Check sheet for the modelled part. Datum: model origin and axes. Units: mm. Round coordinates to 2 decimals unless told otherwise and drop trailing zeros. Loops run counter-clockwise (first coordinate to the right, second up) from the corner with the lowest first, then second, coordinate; pieces in that order, holes last. Notation, with made-up numbers: (27, 87.25) -> (62, 87.25) arc R14 ccw to (62, 106.25) -> close; hole circle Ø4 at (31, 71). An arc over 180 degrees is marked (long way). Return JSON: item names as keys, results as strings.
from build123d import *

# Parameters (mm, degrees)
SKETCH1_W           = 609.6
SKETCH1_H           = 609.6
BOSS_EXTRUDE1_DEPTH = 12.7
SKETCH2_R           = 209.55
CUT_EXTRUDE1_DEPTH  = 13.7
SKETCH3_R           = 19
CUT_EXTRUDE2_DEPTH  = 13.7
SKETCH4_R           = 2.5
CUT_EXTRUDE3_DEPTH  = 13.7
SKETCH5_R           = 3
CUT_EXTRUDE4_DEPTH  = 13.7


with BuildPart() as part:
    # Sketch1 → Boss-Extrude1 (new body)
    with BuildSketch(Plane(origin=(0, 0, 0), x_dir=(1, 0, 0), z_dir=(0, 1, 0))):
        with Locations((254.294265396, -260.340726581)):
            Rectangle(SKETCH1_W, SKETCH1_H)
    extrude(amount=BOSS_EXTRUDE1_DEPTH)

    # Sketch2 → Cut-Extrude1 (cut, through all)
    with BuildSketch(Plane(origin=(0, 12.7, 0), x_dir=(1, 0, 0), z_dir=(0, 1, 0))):
        with Locations((254.294265396, -260.340726581)):
            Circle(SKETCH2_R)
    extrude(amount=-CUT_EXTRUDE1_DEPTH, mode=Mode.SUBTRACT)

    # Sketch3 → Cut-Extrude2 (cut, through all)
    with BuildSketch(Plane.XZ):
        with Locations((489.894265396, 424.740726581)):
            Circle(SKETCH3_R)
    extrude(amount=-CUT_EXTRUDE2_DEPTH, mode=Mode.SUBTRACT)

    # Sketch4 → Cut-Extrude3 (cut, through all)
    with BuildSketch(Plane(origin=(0, 12.7, 0), x_dir=(1, 0, 0), z_dir=(0, 1, 0))):
        with Locations((542.094265396, -355.140726581)):
            Circle(SKETCH4_R)
        with Locations((523.094265396, -348.895728582)):
            Circle(SKETCH4_R)
        with Locations((504.094265396, -342.650730584)):
            Circle(SKETCH4_R)
        with Locations((497.849267397, -361.650730584)):
            Circle(SKETCH4_R)
        with Locations((516.849267397, -367.895728582)):
            Circle(SKETCH4_R)
        with Locations((535.849267397, -374.140726581)):
            Circle(SKETCH4_R)
    extrude(amount=-CUT_EXTRUDE3_DEPTH, mode=Mode.SUBTRACT)

    # Sketch5 → Cut-Extrude4 (cut, through all)
    with BuildSketch(Plane(origin=(0, 12.7, 0), x_dir=(1, 0, 0), z_dir=(0, 1, 0))):
        with Locations((546.394265396, -552.440726581)):
            Circle(SKETCH5_R)
        with Locations((-37.805734604, -552.440726581)):
            Circle(SKETCH5_R)
        with Locations((-37.805734604, 31.759273419)):
            Circle(SKETCH5_R)
        with Locations((546.394265396, 31.759273419)):
            Circle(SKETCH5_R)
    extrude(amount=-CUT_EXTRUDE4_DEPTH, mode=Mode.SUBTRACT)


solid = part.part
Q1. Section check A-A (z = 70). Record the boundary of the cut face in (x, y).
Results list:
{"outline": "(-50.51, 0) -> (166.65, 0) -> (166.65, 12.7) -> (-50.51, 12.7) -> close; (341.94, 0) -> (559.09, 0) -> (559.09, 12.7) -> (341.94, 12.7) -> close"}
Q2. Go/stop test with a flat-tipped pin: pin 1 (5.5 mm diameter, centred on x = 546.39, z = -31.76, fed in from -Y). Record where the tip stops, or that it passes through.
Results list:
{"pin 1": "through"}
Q3. Section check B-B (x = 66.5). Record the boundary of the cut face in (y, z).
Results list:
{"outline": "(0, -44.46) -> (12.7, -44.46) -> (12.7, 167.36) -> (0, 167.36) -> close; (0, 353.32) -> (12.7, 353.32) -> (12.7, 565.14) -> (0, 565.14) -> close"}
Q4. Draft check along X on faces 1 (the cylindrical face through (447.865, 6.439, 340.6)), 2 (the flat face through (182, 0, 53)). Enter one of: released by +X, released by -X, zero draft, split by the parting line, or undercut.
Results list:
{"face 1": "undercut", "face 2": "zero draft"}
Q5. Section check C-C (y = 3.5). Count the separate pieces of the cut face and the enclosed holes in it, then the cut area to 3 significant figures.
Results list:
{"separate pieces": "1", "enclosed holes": "12", "area": "232,000 mm^2"}
Q6. Material ranges on line 1 (X direction, y = 3, z = 268); line 2 (Z direction, x = 252.5, y = 3.75); line 3 (Z direction, x = 67, y = 11), recorded low to high.
Results list:
{"line 1": "-50.51 to 44.88, 463.7 to 559.09", "line 2": "-44.46 to 50.8, 469.88 to 565.14", "line 3": "-44.46 to 166.36, 354.32 to 565.14"}
